Can you work these out from the model? Positions are in its coordinate system, mm. A direction names the side the tool comes from. Give positions to 0.01 mm unless a question says otherwise; leave off trailing zeros. Order: outer loops, then holes, each group sorted by start corner. A loop starts at its lowest first (then second) coordinate and runs counter-clockwise, first axis right, second up.
Item 1: I want a section at D-D, the plane x = 45.1. Write out the boundary of the cut face in (y, z), then the cut area to 3 significant figures.
Item 2: I want a section at A-A, the plane z = 3.8. Write out the boundary of the cut face in (x, y).
Item 3: I want a section at C-C, the plane y = -41.5. Write out the boundary of the cut face in (x, z).
Item 4: If I drill on line 1 along Y through (x, z) = (0.5, 4.25); line 2 along X through (y, z) = (-87, 2); line 3 along Y through (x, z) = (46.5, 4.1) (3 decimals), over which ranges is the centre line in solid material (lowest first)?
Item 5: Which directions (+Z, -Z, +X, -X, +Y, -Y) give clear straight access to the entire face, cutting with the end or side of a thin tool? Please do faces 4 (the flat face through (-11.35, -58, 2)), 5 (the flat face through (40.1, -90, 2)), 6 (the flat face through (16, -113.95, 2)).
Item 6: I'm going to push flat-ended pins straight in: pin 1 Ø2 at (y, z) = (-51.5, 1.5) entering from +X; pin 2 Ø1.3 at (y, z) = (-55.5, 3) entering from +X; pin 3 Ø1.5 at (x, z) = (28, 3) entering from +Y; pin 4 Ø3 at (x, y) = (55.1, -65.45) entering from +Z. Where does each tip first touch, or does it pass through?
Item 7: If we mould it in two halves opening along X, with no side actions, what happens to faces 1 (the flat face through (41, -116.95, 2)), 2 (the flat face through (64.9, -91, 2)), 3 (the cylindrical face through (55.534, -115.902, 2.218))? For each: +X half, -X half, draft (parallel to the pull), parting line (faces both ways), or undercut.
Item 8: I want a section at B-B, the plane x = 0. Write out the boundary of the cut face in (y, z), then the cut area to 3 significant figures.
```python
from build123d import *

# Parameters (mm, degrees)
SKETCH1_R           = 6.35
BOSS_EXTRUDE1_DEPTH = 4.5
SKETCH2_R           = 2
CUT_EXTRUDE1_DEPTH  = 134.826613571
SKETCH3_W           = 5
SKETCH3_H           = 3
CUT_EXTRUDE2_DEPTH  = 134.826613571


with BuildPart() as part:
    # Sketch1 → Boss-Extrude1 (new body)
    with BuildSketch(Plane.XY):
        with BuildLine():
            Line((64.9, -114.9), (64.9, -64.9))
            Line((64.9, -64.9), (9.197116485, 6.650981008))
            ThreePointArc((9.197116485, 6.650981008), (-3.49537036, 10.798374232), (-11.35, 0))
            Line((-11.35, 0), (-11.35, -114.9))
            Line((-11.35, -114.9), (-11.35, -116.95))
            Line((-11.35, -116.95), (35.1, -116.95))
            Line((35.1, -116.95), (64.9, -116.95))
            Line((64.9, -116.95), (64.9, -114.9))
        make_face()
        with BuildLine():
            Line((35.1, -61.9), (35.1, -64.9))
            Line((35.1, -64.9), (35.1, -109.9))
            Line((35.1, -109.9), (-6.35, -109.9))
            Line((-6.35, -109.9), (-6.35, -9.407443861))
            ThreePointArc((-6.35, -9.407443861), (3.681868281, -10.736216557), (10.786933356, -3.530519618))
            Line((10.786933356, -3.530519618), (56.22793669, -61.9))
            Line((56.22793669, -61.9), (35.1, -61.9))
        make_face(mode=Mode.SUBTRACT)
        Polygon((40.1, -69.9), (59.9, -69.9), (59.9, -100), (59.9, -109.9), (50, -109.9), (40.1, -109.9), (40.1, -100), align=None, mode=Mode.SUBTRACT)
        Circle(SKETCH1_R, mode=Mode.SUBTRACT)
    extrude(amount=BOSS_EXTRUDE1_DEPTH)

    # Sketch2 → Cut-Extrude1 (cut, through all)
    with BuildSketch(Plane(origin=(0, 0, 0), x_dir=(-1, 0, 0), z_dir=(0, 0, -1))):
        with Locations((-55.1, -113.95)):
            Circle(SKETCH2_R)
        with Locations((-45.1, -113.95)):
            Circle(SKETCH2_R)
        with Locations((-45.1, -65.45)):
            Circle(SKETCH2_R)
        with Locations((-55.1, -65.45)):
            Circle(SKETCH2_R)
    extrude(amount=-CUT_EXTRUDE1_DEPTH, mode=Mode.SUBTRACT)

    # Sketch3 → Cut-Extrude2 (cut, through all)
    with BuildSketch(Plane.XY.offset(4.5)):
        with Locations((16.15, -115.45)):
            Rectangle(SKETCH3_W, SKETCH3_H)
    extrude(amount=-CUT_EXTRUDE2_DEPTH, mode=Mode.SUBTRACT)


solid = part.part
```
Results list:
1. outline: (-116.95, 0) - (-115.95, 0) - (-115.95, 4.5) - (-116.95, 4.5) - close; (-111.95, 0) - (-109.9, 0) - (-109.9, 4.5) - (-111.95, 4.5) - close; (-69.9, 0) - (-67.45, 0) - (-67.45, 4.5) - (-69.9, 4.5) - close; (-63.45, 0) - (-61.9, 0) - (-61.9, 4.5) - (-63.45, 4.5) - close; (-47.61, 0) - (-39.47, 0) - (-39.47, 4.5) - (-47.61, 4.5) - close
1. area: 68.4 mm2
2. outline: (-11.35, -116.95) - (13.65, -116.95) - (13.65, -113.95) - (18.65, -113.95) - (18.65, -116.95) - (64.9, -116.95) - (64.9, -64.9) - (9.2, 6.65) arc R11.35 ccw to (-11.35, 0) - close; hole (-6.35, -109.9) - (35.1, -109.9) - (35.1, -61.9) - (56.23, -61.9) - (10.79, -3.53) arc R11.35 cw to (-6.35, -9.41) - close; hole circle Ø12.7 at (0, 0); hole (40.1, -109.9) - (59.9, -109.9) - (59.9, -69.9) - (40.1, -69.9) - close; hole circle Ø4 at (45.1, -113.95); hole circle Ø4 at (45.1, -65.45); hole circle Ø4 at (55.1, -113.95); hole circle Ø4 at (55.1, -65.45)
3. outline: (-11.35, 0) - (-6.35, 0) - (-6.35, 4.5) - (-11.35, 4.5) - close; (40.35, 0) - (46.68, 0) - (46.68, 4.5) - (40.35, 4.5) - close
4. line 1: y = -116.95 to -109.9, -11.34 to -6.33, 6.33 to 11.34
4. line 2: x = -11.35 to -6.35, 35.1 to 40.1, 59.9 to 64.9
4. line 3: y = -116.95 to -115.378, -112.522 to -109.9, -69.9 to -66.878, -64.022 to -61.9, -49.404 to -41.265
5. face 4: +Z, -Z, -X, +Y, -Y
5. face 5: +Z, -Z
5. face 6: +Z, -Z, -Y
6. pin 1: stops at x = 55.25
6. pin 2: stops at x = 58.09
6. pin 3: stops at y = -16.54
6. pin 4: passes through
7. face 1: draft
7. face 2: +X half
7. face 3: undercut
8. outline: (-116.95, 0) - (-109.9, 0) - (-109.9, 4.5) - (-116.95, 4.5) - close; (-11.35, 0) - (-6.35, 0) - (-6.35, 4.5) - (-11.35, 4.5) - close; (6.35, 0) - (11.35, 0) - (11.35, 4.5) - (6.35, 4.5) - close
8. area: 76.7 mm2
